Verification items for the finished model (mm, model axes). Coordinates: 2 decimals unless noted, no trailing zeros. Loops run counter-clockwise (first coordinate to the right, second up) from the corner with the lowest first, then second, coordinate; pieces in that order, holes last. Notation, with made-up numbers: (86, -36.5) -> (141, -36.5) arc R20 cw to (141, -17.5) -> close; hole circle Ø9 at (19, 53.5). An arc over 180 degrees is marked (long way). Write item = value, one per line.
```python
from build123d import *

# Parameters (mm, degrees)
BOSS_EXTRUDE1_DEPTH              = 3.175
SKETCH2_R                        = 3.302
CUT_EXTRUDE1_DEPTH               = 3.175
SKETCH4_R                        = 3.302
CUT_EXTRUDE2_DEPTH               = 3.175
F_25_64_0_39063_DIAMETER_HOLE1_D = 9.922002


with BuildPart() as part:
    # Sketch1 → Boss-Extrude1 (new body)
    with BuildSketch(Plane.XY):
        with BuildLine():
            Line((-138.956026155, -36.5125), (-175.156764378, -36.5125))
            ThreePointArc((-175.156764378, -36.5125), (-165.259458004, 74.330287718), (-92.387479089, 158.435905553))
            ThreePointArc((-92.387479089, 158.435905553), (-61.178796261, 170.407509665), (-27.754441861, 170.74473641))
            Line((-27.754441861, 170.74473641), (-72.655722467, 125.843455804))
            ThreePointArc((-72.655722467, 125.843455804), (-131.365317745, 56.585646012), (-136.505752305, -34.06222615))
            Line((-136.505752305, -34.06222615), (-138.956026155, -36.5125))
        make_face()
    extrude(amount=BOSS_EXTRUDE1_DEPTH)

    # Sketch2 → Cut-Extrude1 (cut)
    with BuildSketch(Plane.XY.offset(3.175)):
        with Locations((-142.427155303, 48.347866959)):
            Circle(SKETCH2_R)
        with Locations((-149.837364131, 4.445)):
            Circle(SKETCH2_R)
    extrude(amount=-CUT_EXTRUDE1_DEPTH, mode=Mode.SUBTRACT)

    # Sketch4 → Cut-Extrude2 (cut)
    with BuildSketch(Plane.XY.offset(3.175)):
        with Locations((-164.125827505, 29.433503815)):
            Circle(SKETCH4_R)
        with Locations((-166.205357894, -15.073647178)):
            Circle(SKETCH4_R)
    extrude(amount=-CUT_EXTRUDE2_DEPTH, mode=Mode.SUBTRACT)

    # 25/64 (0.39063) Diameter Hole1 (through all)
    with Locations(Plane.XY.offset(3.175)):
        with Locations((-82.747055002, 138.99473641), (-141.119641567, 90.014320551)):
            Hole(F_25_64_0_39063_DIAMETER_HOLE1_D / 2)


solid = part.part
```
1) Sectioned sample at D-D, the plane x = -106. Record the cut outline in (y, z) (3 decimals), plus the area to 3 significant figures.
Ans:
outline = (97.92, 0) -> (149.329, 0) -> (149.329, 3.175) -> (97.92, 3.175) -> close
area = 163 mm2
2) Sectioned sample at B-B, the plane z = 1.85. Record the cut outline in (x, y) (1 decimal).
Ans:
outline = (-175.2, -36.5) -> (-139, -36.5) -> (-136.5, -34.1) arc R142.9 cw to (-72.7, 125.8) -> (-27.8, 170.7) arc R94.3 ccw to (-92.4, 158.4) arc R181 ccw to start; hole circle Ø6.6 at (-166.2, -15.1); hole circle Ø6.6 at (-164.1, 29.4); hole circle Ø6.6 at (-149.8, 4.4); hole circle Ø9.9 at (-141.1, 90); hole circle Ø6.6 at (-142.4, 48.3); hole circle Ø9.9 at (-82.7, 139)
3) Material ranges on line 1 (Y direction, x = -81, z = 1.55); line 2 (X direction, y = 139, z = 1.1); line 3 (X direction, y = 28, z = 1.05), recorded low to high.
Ans:
line_1 = 120.39 to 134.35, 143.64 to 164.31
line_2 = -118.77 to -87.71, -77.79 to -59.5
line_3 = -178 to -167.1, -161.15 to -139.45
4) Sectioned sample at C-C, the plane y = 155.5. Record the cut outline in (x, z) (3 decimals), plus the area to 3 significant figures.
Ans:
outline = (-97.074, 0) -> (-42.999, 0) -> (-42.999, 3.175) -> (-97.074, 3.175) -> close
area = 172 mm2
5) Depth check by flat-ended pin: pin 1 Ø6 at (x, y) = (-166.21, -15.07) entering from +Z. Enter the tip coordinate at first touch or a pass-through.
Ans:
pin_1 = through
6) Sectioned sample at A-A, the plane x = -84. Record the cut outline in (y, z) (3 decimals).
Ans:
outline = (118.211, 0) -> (134.195, 0) -> (134.195, 3.175) -> (118.211, 3.175) -> close; (143.795, 0) -> (162.952, 0) -> (162.952, 3.175) -> (143.795, 3.175) -> close
7) Release check for a two-part mould opening along X. For faces 1 (the face through (-140.044, 85.171, 1.565)), 2 (the face through (-131, 76, 0)), 3 (the face through (-61.64, 170.32, 1.57)), 4 (the face through (-130.88, 57.78, 1.57)) record: pulls with the +X half, pulls with the -X half, needs draft (parallel to the pull), parting line crosses it, or undercut.
Ans:
face_1 = undercut
face_2 = needs draft
face_3 = parting line crosses it
face_4 = pulls with the +X half
